Autodesk Inventor part; units mm, degrees
ref_plane "YZ Plane" through (0, 0, 0) normal (1, 0, 0) x (0, 1, 0)
ref_plane "XZ Plane" through (0, 0, 0) normal (0, 1, 0) x (-1, 0, 0)
ref_plane "XY Plane" through (0, 0, 0) normal (0, 0, 1) x (1, 0, 0)
sketch "Sketch1" plane through (0, 0, 0) normal (0, 1, 0) x (-1, 0, 0)
  line L0 (76.2, 19.05) -> (-76.2, 19.05)
  line L1 (-76.2, 19.05) -> (-76.2, -19.05)
  line L2 (-76.2, -19.05) -> (76.2, -19.05)
  line L3 (76.2, -19.05) -> (76.2, 19.05)
  line L4 (76.2, 19.05) -> (-76.2, -19.05) construction
  line L5 (-76.2, 19.05) -> (76.2, -19.05) construction
  point P0 (0, 0)
  dimension "d0" = 152.4
  dimension "d1" = 38.1
extrude "Extrusion1" add sketch "Sketch1" along normal blind 5
sketch "Sketch2" plane through (0, 5, 0) normal (0, 1, 0) x (1, 0, 0)
  circle A0 centre (-38.1, 0) radius 6.6
  circle A1 centre (-12.7, 0) radius 6.6
  circle A2 centre (12.7, 0) radius 6.6
  circle A3 centre (38.1, 0) radius 6.6
  line L0 (-76.2, 19.05) -> (-76.2, -19.05)
  line L1 (76.2, -19.05) -> (76.2, 19.05)
  circle A4 centre (-63.5, 0) radius 3.3
  circle A5 centre (63.5, 0) radius 3.3
  point P0 (0, 0)
  dimension "d4" = 13.2
  dimension "d5" = 13.2
  dimension "d6" = 13.2
  dimension "d7" = 13.2
  dimension "d8" = 25.4
  dimension "d9" = 25.4
  dimension "d10" = 25.4
  dimension "d12" = 38.1
  dimension "d13" = 6.6
  dimension "d14" = 6.6
  dimension "d15" = 12.7
  dimension "d16" = 12.7
extrude "Extrusion2" cut sketch "Sketch2" against normal up to next
properties part number "Vial_Plate"
Read the model definition and answer for the solid it produces. Units are mm, in the model's axes. Round coordinates to 2 decimals unless told otherwise and drop trailing zeros. Order: outer loops, then holes, each group sorted by start corner. A loop starts at its lowest first (then second) coordinate and runs counter-clockwise, first axis right, second up. Notation, with made-up numbers: (-6, -32) - (19, -32) arc R5 cw to (19, -23) - close; hole circle Ø5 at (27.5, -26). An arc over 180 degrees is marked (long way). Use one line per item in the form item = value. Start each with the question number.
(1) The part is cut by section A-A (z = 0). Give the vertices of the cut face in (x, y).
(2) Determine the mould class of faces 1 (the face through (76.2, 2, 0)), 2 (the face through (-1, 2, 19.05)), 3 (the face through (-44.694, 2.535, -0.29)) for opening direction Z: +Z half, -Z half, draft (parallel to the pull), parting line (faces both ways), or undercut.
(3) Find the intervals of material crossed by line 1 along Z through (x, y) = (38.1, 3.05); line 2 along Z through (x, y) = (-63.5, 1.2); line 3 along X through (y, z) = (0.7, -4.5), in increasing order. Write a range as from..to.
(4) A flat-ended cylindrical pin translates along its axis: pin 1 Ø12 at (x, z) = (-38.1, 0) entering from +Y. Find the tip coordinate at first contact, or state that the pin passes through.
(5) The part is cut by section B-B (y = 2.15). Give the vertices of the cut face in (x, z).
(6) The part is cut by section C-C (x = -63.5). Give the vertices of the cut face in (y, z), then the cut area to 4 significant figures.
(7) The part is cut by section D-D (x = -12.7). Give the vertices of the cut face in (y, z), then the cut area to 4 significant figures.
Checked values:
q1.outline = (-76.2, 0) - (-66.8, 0) - (-66.8, 5) - (-76.2, 5) - close; (-60.2, 0) - (-44.7, 0) - (-44.7, 5) - (-60.2, 5) - close; (-31.5, 0) - (-19.3, 0) - (-19.3, 5) - (-31.5, 5) - close; (-6.1, 0) - (6.1, 0) - (6.1, 5) - (-6.1, 5) - close; (19.3, 0) - (31.5, 0) - (31.5, 5) - (19.3, 5) - close; (44.7, 0) - (60.2, 0) - (60.2, 5) - (44.7, 5) - close; (66.8, 0) - (76.2, 0) - (76.2, 5) - (66.8, 5) - close
q2.face_1 = draft
q2.face_2 = +Z half
q2.face_3 = undercut
q3.line_1 = -19.05..-6.6, 6.6..19.05
q3.line_2 = -19.05..-3.3, 3.3..19.05
q3.line_3 = -76.2..-42.93, -33.27..-17.53, -7.87..7.87, 17.53..33.27, 42.93..76.2
q4.pin_1 = through
q5.outline = (-76.2, -19.05) - (76.2, -19.05) - (76.2, 19.05) - (-76.2, 19.05) - close; hole circle Ø6.6 at (-63.5, 0); hole circle Ø13.2 at (-38.1, 0); hole circle Ø13.2 at (-12.7, 0); hole circle Ø13.2 at (12.7, 0); hole circle Ø13.2 at (38.1, 0); hole circle Ø6.6 at (63.5, 0)
q6.outline = (0, -19.05) - (5, -19.05) - (5, -3.3) - (0, -3.3) - close; (0, 3.3) - (5, 3.3) - (5, 19.05) - (0, 19.05) - close
q6.area = 157.5 mm^2
q7.outline = (0, -19.05) - (5, -19.05) - (5, -6.6) - (0, -6.6) - close; (0, 6.6) - (5, 6.6) - (5, 19.05) - (0, 19.05) - close
q7.area = 124.5 mm^2
